Source: CAD feature listing. Evaluate the final solid. Frame: model axes, mm. Give positions to 0.01 mm unless a question says otherwise; leave off trailing zeros.
```python
from build123d import *

# Parameters (mm, degrees)
F0_W     = 32
F0_H     = 18
F1_DEPTH = 2208
F3_W     = 32
F3_H     = 32
F4_DEPTH = 2000
F5_W     = 5
F5_H     = 31
F6_DEPTH = 32


with BuildPart() as f1:
    # F0 (on Front) → F1 (new body)
    with BuildSketch(Plane.XZ):
        Rectangle(F0_W, F0_H)
    extrude(amount=F1_DEPTH)

    # F3 (on offset) → F4 (join)
    with BuildSketch(Plane.XZ.offset(50)):
        with Locations((0, 25)):
            Rectangle(F3_W, F3_H)
    extrude(amount=F4_DEPTH)

    # F5 (on face) → F6 (cut)
    with BuildSketch(Plane(origin=(-16, 0, 0), x_dir=(0, -1, 0), z_dir=(-1, 0, 0))):
        with Locations((80.5, 36.5)):
            Rectangle(F5_W, F5_H)
        with Locations((160.5, 36.5)):
            Rectangle(F5_W, F5_H)
        with Locations((240.5, 36.5)):
            Rectangle(F5_W, F5_H)
        with Locations((320.5, 36.5)):
            Rectangle(F5_W, F5_H)
        with Locations((400.5, 36.5)):
            Rectangle(F5_W, F5_H)
        with Locations((480.5, 36.5)):
            Rectangle(F5_W, F5_H)
        with Locations((560.5, 36.5)):
            Rectangle(F5_W, F5_H)
        with Locations((640.5, 36.5)):
            Rectangle(F5_W, F5_H)
        with Locations((720.5, 36.5)):
            Rectangle(F5_W, F5_H)
        with Locations((800.5, 36.5)):
            Rectangle(F5_W, F5_H)
        with Locations((880.5, 36.5)):
            Rectangle(F5_W, F5_H)
        with Locations((960.5, 36.5)):
            Rectangle(F5_W, F5_H)
        with Locations((1040.5, 36.5)):
            Rectangle(F5_W, F5_H)
        with Locations((1120.5, 36.5)):
            Rectangle(F5_W, F5_H)
        with Locations((1200.5, 36.5)):
            Rectangle(F5_W, F5_H)
        with Locations((1280.5, 36.5)):
            Rectangle(F5_W, F5_H)
        with Locations((1360.5, 36.5)):
            Rectangle(F5_W, F5_H)
        with Locations((1440.5, 36.5)):
            Rectangle(F5_W, F5_H)
        with Locations((1520.5, 36.5)):
            Rectangle(F5_W, F5_H)
        with Locations((1600.5, 36.5)):
            Rectangle(F5_W, F5_H)
        with Locations((1680.5, 36.5)):
            Rectangle(F5_W, F5_H)
        with Locations((1760.5, 36.5)):
            Rectangle(F5_W, F5_H)
        with Locations((1840.5, 36.5)):
            Rectangle(F5_W, F5_H)
        with Locations((1920.5, 36.5)):
            Rectangle(F5_W, F5_H)
        with Locations((2000.5, 36.5)):
            Rectangle(F5_W, F5_H)
    extrude(amount=-F6_DEPTH, mode=Mode.SUBTRACT)


solid = f1.part
```
1) Section query A-A, the plane z = 29. Count the separate pieces of the cut face and the enclosed holes in it, and give its area (3 significant figures).
Report:
separate pieces: 26
enclosed holes: 0
area: 60,000 mm2
2) Material intervals for L1, parallel to Y at x = -12, z = 9.5, sorted ascending.
Report:
L1: y = -2050 to -50
3) Pin query (flat end, axial travel): pin 1 (6 mm diameter, centred on x = -6.5, z = 27, fed in from -Y); pin 2 (16 mm diameter, centred on x = 2.5, z = 31, fed in from +Y); pin 3 (2.5 mm diameter, centred on x = 1, y = -561.5, fed in from +Z). Return the tip coordinate at first contact, or that it passes through.
Report:
pin 1: stops at y = -2050
pin 2: stops at y = -50
pin 3: stops at z = 21
